from build123d import *

# Parameters (mm, degrees)
SKETCH2_W           = 43.18
SKETCH2_H           = 10.16
BOSS_EXTRUDE1_DEPTH = 2.54
SKETCH3_W           = 38.1
SKETCH3_H           = 3.81
BOSS_EXTRUDE2_DEPTH = 6.35
SKETCH4_R           = 1.143
CUT_EXTRUDE1_DEPTH  = 24.070695698
BOSS_EXTRUDE3_DEPTH = 38.1
SKETCH6_R           = 1.25
CUT_EXTRUDE2_DEPTH  = 26.677507073


with BuildPart() as part:
    # Sketch2 → Boss-Extrude1 (new body)
    with BuildSketch(Plane(origin=(0, 0, 0), x_dir=(1, 0, 0), z_dir=(0, 1, 0))):
        Rectangle(SKETCH2_W, SKETCH2_H)
    extrude(amount=BOSS_EXTRUDE1_DEPTH)

    # Sketch3 → Boss-Extrude2 (add)
    with BuildSketch(Plane(origin=(0, 2.54, 0), x_dir=(1, 0, 0), z_dir=(0, 1, 0))):
        with Locations((0, -3.175)):
            Rectangle(SKETCH3_W, SKETCH3_H)
    extrude(amount=BOSS_EXTRUDE2_DEPTH)

    # Sketch4 → Cut-Extrude1 (cut, through all)
    with BuildSketch(Plane(origin=(0, 2.54, 0), x_dir=(1, 0, 0), z_dir=(0, 1, 0))):
        with Locations(Location((19.05, 1.905, 0), (0, 0, 270))):
            Circle(SKETCH4_R)
        with Locations(Location((-19.05, 1.905, 0), (0, 0, 270))):
            Circle(SKETCH4_R)
    extrude(amount=-CUT_EXTRUDE1_DEPTH, mode=Mode.SUBTRACT)

    # Sketch5 → Boss-Extrude3 (add)
    with BuildSketch(Plane.ZY.offset(19.05)):
        Polygon((5.08, 8.89), (6.329408021, 8.89), (5.08, 0), align=None)
    extrude(amount=-BOSS_EXTRUDE3_DEPTH)

    # Sketch6 → Cut-Extrude2 (cut, through all)
    with BuildSketch(Plane(origin=(0, -0.700118884, 4.981604708), x_dir=(1, 0, 0), z_dir=(0, -0.1391731009600584, 0.9902680687415715))):
        with Locations(Location((-16.51, 5.195682913, 0), (0, 0, 270))):
            Circle(SKETCH6_R)
        with Locations(Location((16.51, 5.195682913, 0), (0, 0, 270))):
            Circle(SKETCH6_R)
    extrude(amount=-CUT_EXTRUDE2_DEPTH, mode=Mode.SUBTRACT)


solid = part.part
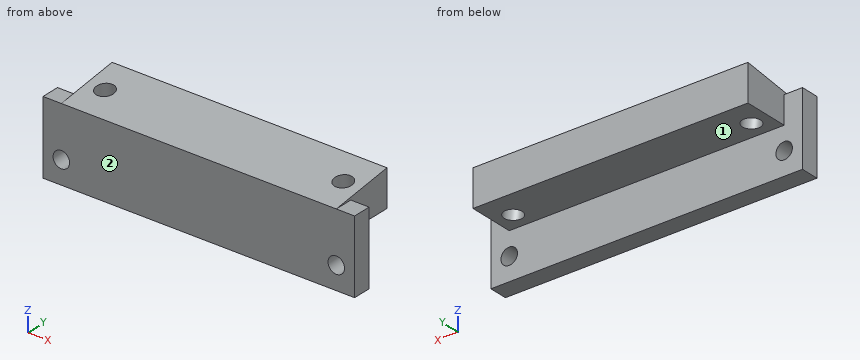
Read the model definition and answer for the solid it produces. Units are mm, in the model's axes. Face numbers are marked on the shaded views. A direction names the side the tool comes from. Coordinates: 2 decimals unless noted, no trailing zeros. Write each loop counter-clockwise with the first axis right and the second up, starting at its lowest first coordinate (ties: lowest second). Pieces come first, ordered by that corner, then holes. Notation, with made-up numbers: M 84.25,23.25 L 129.25,23.25 A36 cw 129.25,57.25 Z; hole C -22.75,-38.5 d9. An arc over 180 degrees is marked long. Use a Markdown table: item, result.
Q1. The part is cut by section A-A, the plane x = -11. Write down the section's boundary in (y, z).
Answer block:
| item | result |
|---|---|
| outline | M 0,-5.08 L 2.54,-5.08 L 2.54,1.27 L 8.89,1.27 L 8.89,6.33 L 0,5.08 Z |
Q2. Straight lines are drawn through the part: L1, parallel to X at y = 4, z = 5.25; L2, parallel to X at y = 4.25, z = 2; L3, parallel to Y at x = 13.5, z = -1. For each, find the intervals that lie inside material, in ascending order. Write a range as [from, to].
Answer block:
| item | result |
|---|---|
| L1 | x = [-19.05, -17.65], [-15.37, 15.37], [17.65, 19.05] |
| L2 | x = [-19.05, -17.54], [-15.48, 15.48], [17.54, 19.05] |
| L3 | y = [0, 2.54] |
Q3. The part is cut by section C-C, the plane y = 5.5. Give the number of separate pieces and of enclosed holes in the cut face, then the cut area to 3 significant figures.
Answer block:
| item | result |
|---|---|
| separate pieces | 3 |
| enclosed holes | 0 |
| area | 157 mm2 |
Q4. Each of these flat-tipped pins is pushed along its axis until it touches: pin 1 Ø1.8 at (x, z) = (-19.05, -1.905) entering from -Y; pin 2 Ø1.5 at (y, z) = (5, 3.5) entering from -X; pin 3 Ø1.3 at (x, y) = (20, 1.5) entering from +Z; pin 4 Ø3 at (x, z) = (19.05, -1.905) entering from +Y. Where does it stop, or does it pass through?
Answer block:
| item | result |
|---|---|
| pin 1 | passes through |
| pin 2 | stops at x = -19.05 |
| pin 3 | stops at z = 5.08 |
| pin 4 | stops at y = 2.54 |
Q5. The part is cut by section B-B, the plane y = 1. Write down the section's boundary in (x, z) (3 decimals), then the cut area to 3 significant figures.
Answer block:
| item | result |
|---|---|
| outline | M -21.59,-5.08 L 21.59,-5.08 L 21.59,5.08 L 19.05,5.08 L 19.05,5.221 L -19.05,5.221 L -19.05,5.08 L -21.59,5.08 Z; hole C -19.05,-1.905 d2.286; hole C 19.05,-1.905 d2.286 |
| area | 436 mm2 |
Q6. Which of the six approach directions +Z, -Z, +X, -X, +Y, -Y give full straight-line access (tool end or side, diameter ignored) to the marked faces 1 and 2?
Answer block:
| item | result |
|---|---|
| face 1 | -Z, +X, -X, +Y |
| face 2 | +Z, -Z, +X, -X, -Y |
